Part print with two shaded views. Sizes in mm from the minimum x, y, z corner. Round coordinates to 2 decimals unless told otherwise and drop trailing zeros. Order: outer loops, then holes, each group sorted by start corner. A loop starts at its lowest first (then second) coordinate and runs counter-clockwise, first axis right, second up. Notation, with made-up numbers: M -14,74 L 14,74 A11 cw 14,83 Z; hole C 35.25,86 d7. An arc over 180 degrees is marked long. Answer as a JSON object with one key per item and string values.
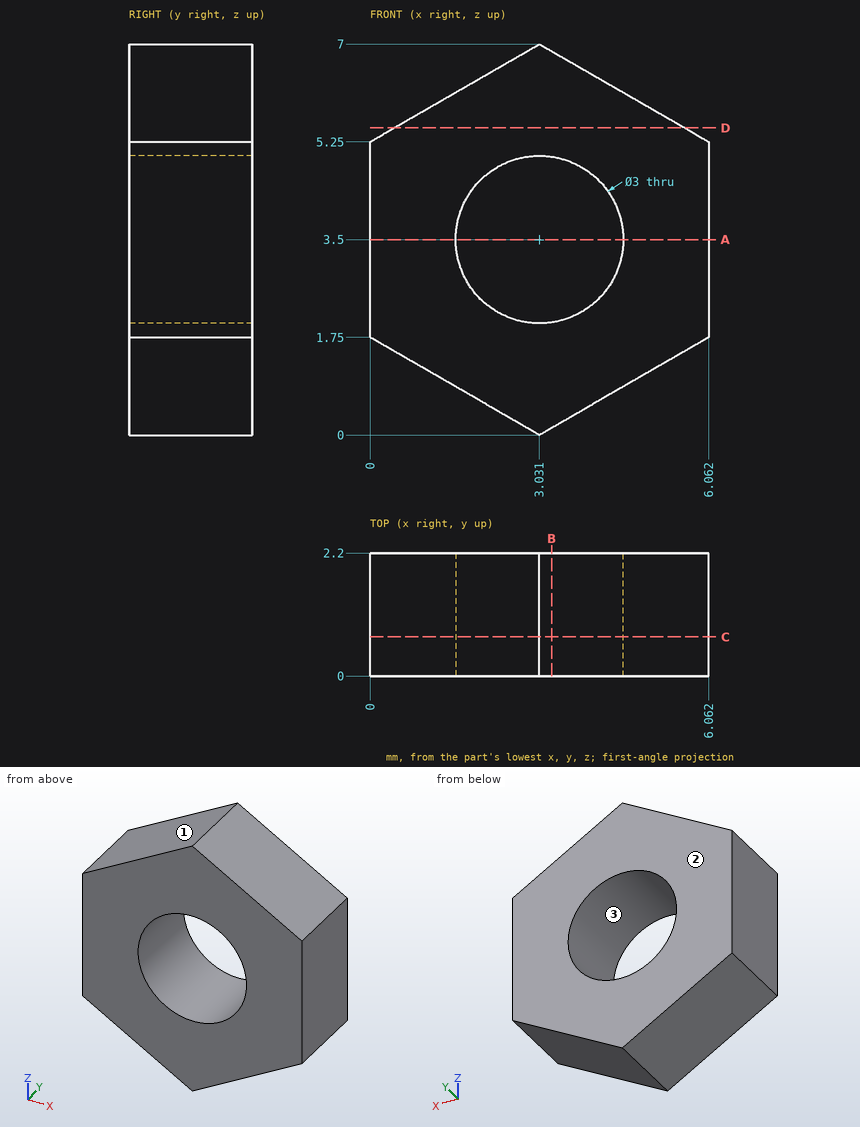
Item 1: Saw through at A-A on z = 3.5. List the corners of the cut face in (x, y).
Worked answers:
{"outline": "M 0,0 L 1.53,0 L 1.53,2.2 L 0,2.2 Z; M 4.53,0 L 6.06,0 L 6.06,2.2 L 4.53,2.2 Z"}
Item 2: Saw through at B-B on x = 3.25. List the corners of the cut face in (y, z).
Worked answers:
{"outline": "M 0,0.13 L 2.2,0.13 L 2.2,2.02 L 0,2.02 Z; M 0,4.98 L 2.2,4.98 L 2.2,6.87 L 0,6.87 Z"}
Item 3: Saw through at D-D on z = 5.5. List the corners of the cut face in (x, y), and give its area (3 significant figures).
Worked answers:
{"outline": "M 0.43,0 L 5.63,0 L 5.63,2.2 L 0.43,2.2 Z", "area": "11.4 mm2"}
Item 4: Wall check: line 1 along X through (y, z) = (0.8, 3.5); line 2 along Z through (x, y) = (3.25, 2.1); line 3 along X through (y, z) = (2.1, 3) (1 decimal). Give the ranges that are in metal, low to high. Write a range as [from, to].
Worked answers:
{"line 1": "x = [0, 1.53], [4.53, 6.06]", "line 2": "z = [0.13, 2.02], [4.98, 6.87]", "line 3": "x = [0, 1.6], [4.4, 6.1]"}
Item 5: Saw through at C-C on y = 0.7. List the corners of the cut face in (x, z).
Worked answers:
{"outline": "M 0,1.75 L 3.03,0 L 6.06,1.75 L 6.06,5.25 L 3.03,7 L 0,5.25 Z; hole C 3.03,3.5 d3"}
Item 6: Two-plate mould, pull along X, no slides. Class the marked faces 1, 2 and 3: released by +X, released by -X, zero draft, split by the parting line, or undercut.
Worked answers:
{"face 1": "released by -X", "face 2": "zero draft", "face 3": "undercut"}
